```python
from build123d import *

# Parameters (mm, degrees)
BOSS_EXTRUDE1_DEPTH       = 3.175
FILLET1_R                 = 5
F_6_32_TAPPED_HOLE1_D     = 2.7051
F_6_32_TAPPED_HOLE1_DEPTH = 10.973
F_6_32_TAPPED_HOLE1_TIP   = 0.81269403
FILLET2_R                 = 5


with BuildPart() as part:
    # Sketch2 → Boss-Extrude1 (new body)
    with BuildSketch(Plane.XY):
        Polygon((0, 24.784092681), (24.784092681, 0), (0, -24.784092681), (-24.784092681, 0), align=None)
        Polygon((0, 13.470384182), (13.470384182, 0), (0, -13.470384182), (-13.470384182, 0), align=None, mode=Mode.SUBTRACT)
    extrude(amount=BOSS_EXTRUDE1_DEPTH)

    # Fillet1
    fillet1_edges = [part.edges().sort_by_distance(p)[0] for p in [
        (0, 13.470384182, 1.5875),
        (-13.470384182, 0, 1.5875),
        (0, -13.470384182, 1.5875),
        (13.470384182, 0, 1.5875),
    ]]
    fillet(fillet1_edges, radius=FILLET1_R)

    # #6-32 Tapped Hole1
    with Locations(Plane(origin=(0, 0, 0), x_dir=(-1, 0, 0), z_dir=(0, 0, -1))):
        with Locations((-18, 0), (0, 18), (0, -18), (18, 0)):
            Hole(F_6_32_TAPPED_HOLE1_D / 2, depth=F_6_32_TAPPED_HOLE1_DEPTH)
            with Locations((0, 0, -(F_6_32_TAPPED_HOLE1_DEPTH + F_6_32_TAPPED_HOLE1_TIP / 2))):  # 118° drill point
                Cone(0, F_6_32_TAPPED_HOLE1_D / 2, F_6_32_TAPPED_HOLE1_TIP, mode=Mode.SUBTRACT)

    # Fillet2
    fillet2_edges = [part.edges().sort_by_distance(p)[0] for p in [
        (0, 24.784092681, 1.5875),
        (24.784092681, 0, 1.5875),
        (0, -24.784092681, 1.5875),
        (-24.784092681, 0, 1.5875),
    ]]
    fillet(fillet2_edges, radius=FILLET2_R)


solid = part.part
```
Read the model definition and answer for the solid it produces. Units are mm, in the model's axes. A direction names the side the tool comes from. Coordinates: 2 decimals unless noted, no trailing zeros. Order: outer loops, then holes, each group sorted by start corner. A loop starts at its lowest first (then second) coordinate and runs counter-clockwise, first axis right, second up. Notation, with made-up numbers: (-23.5, -25.75) - (30.5, -25.75) arc R26 ccw to (30.5, 10.25) - close; hole circle Ø5 at (16.5, -9.5). An arc over 180 degrees is marked (long way). Answer as a JSON object with one key per item and string values. Group by question number.
Item 1: A tool of negligible diameter and unlimited length cuts with its end or side. For faces 1 (the face through (-10, -5, 0)), 2 (the face through (-6.78, 6.69, 1.57)), from which of +Z, -Z, +X, -X, +Y, -Y can it reach the whole face along a straight path? Write none if from no direction.
Item 2: Section D-D (y = -18) is taken. Give the vertices of the cut face in (x, z) (3 decimals), plus the area to 3 significant figures.
Item 3: Consider probe 1 along Y at (x, z) = (0, 0.9); probe 2 along X at (y, z) = (1, 1.9); probe 3 along Y at (x, z) = (18, 1.7). Determine where each line is inside the solid, lowest interval first. Write a range as from..to.
Item 4: Flat-ended cylindrical pins translate along their axes: P1, Ø2, axis at x = 18, y = 0, coming from the -Z side; P2, Ø1, axis at x = 13.5, z = 2.5, coming from the -Y side; P3, Ø1.5, axis at x = 10, z = 1.5, coming from the -Y side. Find the tip coordinate at first contact, or state that the pin passes through.
Item 5: Section C-C (z = 1.7) is taken. Give the vertices of the cut face in (x, y), plus the area to 3 significant figures.
Item 6: The mould has two halves that part along X. Classify faces 3 (the face through (0.055, -22.713, 1.61)), 4 (the face through (6.78, -6.69, 1.57)), 5 (the face through (-6.69, -6.78, 1.57)), 6 (the face through (12.268, 12.516, 1.565)): +X half, -X half, draft (parallel to the pull), parting line (faces both ways), or undercut.
Item 7: Section A-A (x = 0) is taken. Give the vertices of the cut face in (y, z) (3 decimals).
Results are:
{
 "1": {"face 1": "-Z, +X, -X, +Y, -Y", "face 2": "+Z, -Z"},
 "2": {"outline": "(-6.784, 0) - (-1.353, 0) - (-1.353, 3.175) - (-6.784, 3.175) - close; (1.353, 0) - (6.784, 0) - (6.784, 3.175) - (1.353, 3.175) - close", "area": "34.5 mm^2"},
 "3": {"probe 1": "y = -22.71..-19.35, -16.65..-11.4, 11.4..16.65, 19.35..22.71", "probe 2": "x = -22.61..-18.91, -17.09..-11.3, 11.3..17.09, 18.91..22.61", "probe 3": "y = -6.78..-1.35, 1.35..6.78"},
 "4": {"P1": "passes through", "P2": "stops at y = -11.78", "P3": "stops at y = -15.53"},
 "5": {"outline": "(-21.25, -3.54) - (-3.54, -21.25) arc R5 ccw to (3.54, -21.25) - (21.25, -3.54) arc R5 ccw to (21.25, 3.54) - (3.54, 21.25) arc R5 ccw to (-3.54, 21.25) - (-21.25, 3.54) arc R5 ccw to start; hole circle Ø2.71 at (-18, 0); hole (-9.93, -3.54) - (-3.54, -9.93) arc R5 ccw to (3.54, -9.93) - (9.93, -3.54) arc R5 ccw to (9.93, 3.54) - (3.54, 9.93) arc R5 ccw to (-3.54, 9.93) - (-9.93, 3.54) arc R5 ccw to start; hole circle Ø2.71 at (0, -18); hole circle Ø2.71 at (0, 18); hole circle Ø2.71 at (18, 0)", "area": "843 mm^2"},
 "6": {"face 3": "parting line", "face 4": "undercut", "face 5": "undercut", "face 6": "+X half"},
 "7": {"outline": "(-22.713, 0) - (-19.353, 0) - (-19.353, 3.175) - (-22.713, 3.175) - close; (-16.647, 0) - (-11.399, 0) - (-11.399, 3.175) - (-16.647, 3.175) - close; (11.399, 0) - (16.647, 0) - (16.647, 3.175) - (11.399, 3.175) - close; (19.353, 0) - (22.713, 0) - (22.713, 3.175) - (19.353, 3.175) - close"}
}
